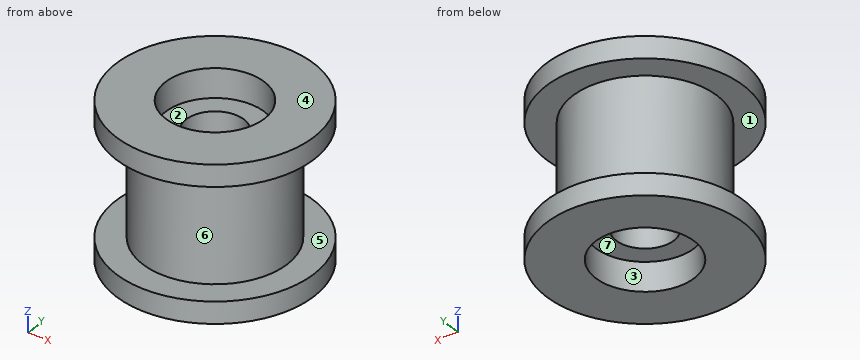
Autodesk Inventor part; units mm, degrees
ref_plane "YZ Plane" through (0, 0, 0) normal (1, 0, 0) x (0, 1, 0)
ref_plane "XZ Plane" through (0, 0, 0) normal (0, 1, 0) x (-1, 0, 0)
ref_plane "XY Plane" through (0, 0, 0) normal (0, 0, 1) x (1, 0, 0)
sketch "Base" plane through (0, 0, 0) normal (0, 0, 1) x (1, 0, 0)
  circle A0 centre (0, 0) radius 10.25
  dimension "d0" = 20.5
extrude "BaseFeature" add sketch "Base" along normal mid plane 16
sketch "Ridges" plane through (0, 0, 0) normal (0, 0, 1) x (1, 0, 0)
  circle A0 centre (0, 0) radius 10.25
  circle A1 centre (0, 0) radius 7.5
  dimension "d3" = 15
extrude "RidgesFeature" cut sketch "Ridges" along normal mid plane 11.5
sketch "Countersink" plane through (0, 0, 8) normal (0, 0, 1) x (1, 0, 0)
  circle A0 centre (0, 0) radius 5.125
  dimension "d6" = 10.25
extrude "CountersinkFeature" cut sketch "Countersink" against normal blind 3
mirror "CountersinkMirrorFeature" about plane through (0, 0, 0) normal (0, 0, 1) of "CountersinkFeature"
sketch "MountHole" plane through (0, 0, 5) normal (0, 0, 1) x (1, 0, 0)
  point P0 (0, 0)
hole "MountHoleFeature" at (0, 0, 5) direction (0, 0, -1) diameter 6 end through all
properties part number "LegChainTensionerBlock"
Check sheet for the modelled part. Datum: model origin and axes. Units: mm. Face numbers are marked on the shaded views. A direction names the side the tool comes from. Round coordinates to 2 decimals unless told otherwise and drop trailing zeros. Write each loop counter-clockwise with the first axis right and the second up, starting at its lowest first coordinate (ties: lowest second). Pieces come first, ordered by that corner, then holes. Notation, with made-up numbers: M 8.5,-31 L 25.5,-31 A25 cw 25.5,-11 Z; hole C 56.5,-4.75 d7. An arc over 180 degrees is marked long. Write item = value, one per line. Start each with the question number.
1. Section check C-C, the plane z = 0.75. Record the cut outline in (x, y), then the cut area to 3 significant figures.
2. Scan lines: line 1 (Z direction, x = 6.5, y = 4.5); line 2 (Y direction, x = 0, z = -3.25); line 3 (Y direction, x = 0, z = -6.6) (3 decimals). Record each from-to range of solid material in increasing order. Write a range as [from, to].
3. Gauge pin test, flat ends, axial feed: pin 1 (8 mm diameter, centred on x = 0, y = 0, fed in from -Z); pin 2 (3 mm diameter, centred on x = 2.5, y = 2.5, fed in from +Z); pin 3 (8 mm diameter, centred on x = 5, z = -1.5, fed in from -Y); pin 4 (1 mm diameter, centred on x = -0.5, y = -0.5, fed in from +Z). Record the tip position at first contact, or that the pin passes through.
4. Section check D-D, the plane x = 4.5. Record the cut outline in (y, z), then the cut area to 3 significant figures.
5. Tool access check on the marked faces 1, 2, 3 and 4. Record the directions out of +Z, -Z, +X, -X, +Y, -Y that give a thin tool (end or side, any length) a straight path to the whole face; none if there is none.
6. Release check for a two-part mould opening along X. For the marked faces 5, 6 and 7 record: pulls with the +X half, pulls with the -X half, needs draft (parallel to the pull), parting line crosses it, or undercut.
7. Section check A-A, the plane x = 0. Record the cut outline in (y, z) (3 decimals).
Results found:
q1.outline = C 0,0 d15; hole C 0,0 d6
q1.area = 148 mm^2
q2.line_1 = [-8, -5.75], [5.75, 8]
q2.line_2 = [-7.5, -3], [3, 7.5]
q2.line_3 = [-10.25, -5.125], [5.125, 10.25]
q3.pin_1 = -5
q3.pin_2 = 5
q3.pin_3 = -7.43
q3.pin_4 = through
q4.outline = M -9.21,-8 L -2.45,-8 L -2.45,-5 L 2.45,-5 L 2.45,-8 L 9.21,-8 L 9.21,-5.75 L 6,-5.75 L 6,5.75 L 9.21,5.75 L 9.21,8 L 2.45,8 L 2.45,5 L -2.45,5 L -2.45,8 L -9.21,8 L -9.21,5.75 L -6,5.75 L -6,-5.75 L -9.21,-5.75 Z
q4.area = 191 mm^2
q5.face_1 = none
q5.face_2 = +Z
q5.face_3 = -Z
q5.face_4 = +Z, +X, -X, +Y, -Y
q6.face_5 = needs draft
q6.face_6 = parting line crosses it
q6.face_7 = undercut
q7.outline = M -10.25,-8 L -5.125,-8 L -5.125,-5 L -3,-5 L -3,5 L -5.125,5 L -5.125,8 L -10.25,8 L -10.25,5.75 L -7.5,5.75 L -7.5,-5.75 L -10.25,-5.75 Z; M 3,-5 L 5.125,-5 L 5.125,-8 L 10.25,-8 L 10.25,-5.75 L 7.5,-5.75 L 7.5,5.75 L 10.25,5.75 L 10.25,8 L 5.125,8 L 5.125,5 L 3,5 Z
